from build123d import *

# Parameters (mm, degrees)
BOSS_EXTRUDE3_DEPTH      = 3.249999
BOSS_EXTRUDE3_DEPTH_BACK = 16.581442
SKETCH1_W                = 34.3
SKETCH1_H                = 66.5
CUT_EXTRUDE1_DEPTH       = 5
CUT_EXTRUDE2_DEPTH       = 5
FILLET1_R                = 2
SKETCH5_W                = 51.30778099
SKETCH5_H                = 76.39990746
CUT_EXTRUDE3_DEPTH       = 14
SKETCH6_W                = 31.3
SKETCH6_H                = 63.5
CUT_EXTRUDE4_DEPTH       = 4.831437303
SKETCH7_W                = 26.3
SKETCH7_H                = 4
SKETCH7_W_2              = 25.3
BOSS_EXTRUDE4_DEPTH      = 9.5
SKETCH8_W                = 20.3
SKETCH8_H                = 55.5
BOSS_EXTRUDE5_DEPTH      = 2
CUT_EXTRUDE5_DEPTH       = 1.5


with BuildPart() as part:
    # Sketch1 → Boss-Extrude3 (new, two sides: drawn at the far end of the back side and taken through both)
    with BuildSketch(Plane.XY.offset(-BOSS_EXTRUDE3_DEPTH_BACK)):
        with Locations((-15.15, 31.25)):
            Rectangle(SKETCH1_W, SKETCH1_H)
    extrude(amount=BOSS_EXTRUDE3_DEPTH + BOSS_EXTRUDE3_DEPTH_BACK)

    # Sketch3 → Cut-Extrude1 (cut)
    with BuildSketch(Plane.ZY.offset(32.3)):
        with BuildLine():
            Line((-13.946442816, 47.860002379), (-13.946442816, 14.260002379))
            add(Edge.make_bspline(
                [(-13.946442816, 14.260002379), (-13.946442816, 14.019317473), (-13.90167089, 13.549905983), (-13.594210712, 12.544215416), (-12.741245974, 11.38215204), (-11.448721179, 10.74393594), (-10.404919412, 10.615783107), (-9.934864774, 10.653203818), (-9.697836412, 10.694998313)],
                knots=[0, 0, 0, 0, 0.125, 0.25, 0.5, 0.75, 0.875, 1, 1, 1, 1], degree=3))
            Line((-9.697836412, 10.694998313), (-6.707836413, 11.222215985))
            add(Edge.make_bspline(
                [(-6.707836413, 11.222215985), (-6.30796959, 11.292723295), (-5.54451734, 11.557407058), (-4.497780226, 12.405299319), (-3.844533346, 13.58336909), (-3.716442816, 14.381184638), (-3.716442816, 14.787220052)],
                knots=[0, 0, 0, 0, 0.25, 0.5, 0.75, 1, 1, 1, 1], degree=3))
            Line((-3.716442816, 14.787220052), (-3.716442816, 47.332784706))
            add(Edge.make_bspline(
                [(-3.716442816, 47.332784706), (-3.716442815, 47.73882012), (-3.844533346, 48.536635667), (-4.497780225, 49.714705439), (-5.544517339, 50.5625977), (-6.307969589, 50.827281463), (-6.707836412, 50.897788773)],
                knots=[0, 0, 0, 0, 0.25, 0.5, 0.75, 1, 1, 1, 1], degree=3))
            Line((-6.707836412, 50.897788773), (-9.697836412, 51.425006445))
            add(Edge.make_bspline(
                [(-9.697836412, 51.425006445), (-9.934864773, 51.46680094), (-10.404919411, 51.504221651), (-11.448721179, 51.376068818), (-12.741245974, 50.737852719), (-13.594210712, 49.575789343), (-13.90167089, 48.570098776), (-13.946442816, 48.100687285), (-13.946442816, 47.860002379)],
                knots=[0, 0, 0, 0, 0.125, 0.25, 0.5, 0.75, 0.875, 1, 1, 1, 1], degree=3))
        make_face()
    extrude(amount=-CUT_EXTRUDE1_DEPTH, mode=Mode.SUBTRACT)

    # Sketch4 → Cut-Extrude2 (cut)
    with BuildSketch(Plane(origin=(2, 0, 0), x_dir=(0, 0, -1), z_dir=(1, 0, 0))):
        with BuildLine():
            Line((6.817836087, 38.212213104), (9.807836086, 37.684995431))
            add(Edge.make_bspline(
                [(9.807836086, 37.684995431), (10.044864448, 37.643200936), (10.514919086, 37.605780225), (11.558720853, 37.733933058), (12.851245648, 38.372149158), (13.704210386, 39.534212534), (14.011670565, 40.539903101), (14.05644249, 41.009314591), (14.05644249, 41.249999497)],
                knots=[0, 0, 0, 0, 0.125, 0.25, 0.5, 0.75, 0.875, 1, 1, 1, 1], degree=3))
            Line((14.05644249, 41.249999497), (14.05644249, 52.799999497))
            add(Edge.make_bspline(
                [(14.05644249, 52.799999497), (14.05644249, 53.040684403), (14.011670565, 53.510095894), (13.704210386, 54.51578646), (12.851245648, 55.677849837), (11.558720853, 56.316065936), (10.514919086, 56.444218769), (10.044864448, 56.406798058), (9.807836087, 56.365003563)],
                knots=[0, 0, 0, 0, 0.125, 0.25, 0.5, 0.75, 0.875, 1, 1, 1, 1], degree=3))
            Line((9.807836087, 56.365003563), (6.817836087, 55.837785891))
            add(Edge.make_bspline(
                [(6.817836087, 55.837785891), (6.417969263, 55.767278581), (5.654517014, 55.502594818), (4.6077799, 54.654702557), (3.95453302, 53.476632786), (3.82644249, 52.678817239), (3.82644249, 52.272781825)],
                knots=[0, 0, 0, 0, 0.25, 0.5, 0.75, 1, 1, 1, 1], degree=3))
            Line((3.82644249, 52.272781825), (3.82644249, 41.77721717))
            add(Edge.make_bspline(
                [(3.82644249, 41.77721717), (3.82644249, 41.371181756), (3.95453302, 40.573366208), (4.6077799, 39.395296437), (5.654517014, 38.547404177), (6.417969263, 38.282720413), (6.817836087, 38.212213104)],
                knots=[0, 0, 0, 0, 0.25, 0.5, 0.75, 1, 1, 1, 1], degree=3))
        make_face()
        with BuildLine():
            Line((3.82644249, 20.772783732), (3.82644249, 10.277219077))
            add(Edge.make_bspline(
                [(3.82644249, 10.277219077), (3.82644249, 9.871183663), (3.95453302, 9.073368116), (4.6077799, 7.895298345), (5.654517014, 7.047406084), (6.417969263, 6.782722321), (6.817836087, 6.712215011)],
                knots=[0, 0, 0, 0, 0.25, 0.5, 0.75, 1, 1, 1, 1], degree=3))
            Line((6.817836087, 6.712215011), (9.807836086, 6.184997339))
            add(Edge.make_bspline(
                [(9.807836086, 6.184997339), (10.044864448, 6.143202843), (10.514919086, 6.105782132), (11.558720853, 6.233934965), (12.851245648, 6.872151065), (13.704210386, 8.034214441), (14.011670565, 9.039905008), (14.05644249, 9.509316499), (14.05644249, 9.750001404)],
                knots=[0, 0, 0, 0, 0.125, 0.25, 0.5, 0.75, 0.875, 1, 1, 1, 1], degree=3))
            Line((14.05644249, 9.750001404), (14.05644249, 21.300001404))
            add(Edge.make_bspline(
                [(14.05644249, 21.300001404), (14.05644249, 21.54068631), (14.011670565, 22.010097801), (13.704210386, 23.015788368), (12.851245648, 24.177851744), (11.558720853, 24.816067843), (10.514919086, 24.944220677), (10.044864448, 24.906799966), (9.807836087, 24.86500547)],
                knots=[0, 0, 0, 0, 0.125, 0.25, 0.5, 0.75, 0.875, 1, 1, 1, 1], degree=3))
            Line((9.807836087, 24.86500547), (6.817836087, 24.337787798))
            add(Edge.make_bspline(
                [(6.817836087, 24.337787798), (6.417969263, 24.267280488), (5.654517014, 24.002596725), (4.6077799, 23.154704464), (3.95453302, 21.976634693), (3.82644249, 21.178819146), (3.82644249, 20.772783732)],
                knots=[0, 0, 0, 0, 0.25, 0.5, 0.75, 1, 1, 1, 1], degree=3))
        make_face()
    extrude(amount=-CUT_EXTRUDE2_DEPTH, mode=Mode.SUBTRACT)

    # Fillet1
    fillet1_edges = [part.edges().sort_by_distance(p)[0] for p in [
        (-32.3, -2, -6.6657215),
        (2, -2, -6.6657215),
        (2, 64.5, -6.6657215),
        (-32.3, 64.5, -6.6657215),
    ]]
    fillet(fillet1_edges, radius=FILLET1_R)

    # Sketch5 → Cut-Extrude3 (cut)
    with BuildSketch(Plane(origin=(0, 2.84e-07, 3.250003097), x_dir=(1, 0, 0), z_dir=(0, 8.742273400000003e-08, 0.9999999999999963))):
        with Locations((-12.815688561, 29.564706803)):
            Rectangle(SKETCH5_W, SKETCH5_H)
    extrude(amount=-CUT_EXTRUDE3_DEPTH, mode=Mode.SUBTRACT)


with BuildPart() as cut_extrude3_kept_piece:
    # of the separate pieces the step leaves, the one the design keeps (cut_extrude3_pieces_kept)
    add(part.part.solids().sort_by_distance((-30.3, 64.5, -16.581442))[0])

    # Sketch6 → Cut-Extrude4 (cut)
    with BuildSketch(Plane(origin=(0, -9.4e-07, -10.749996903), x_dir=(1, 0, 0), z_dir=(0, 8.742273399652584e-08, 0.9999999999999963))):
        with Locations((-15.15, 31.25000094)):
            Rectangle(SKETCH6_W, SKETCH6_H)
    extrude(amount=-CUT_EXTRUDE4_DEPTH, mode=Mode.SUBTRACT)


with BuildPart() as boss_extrude4_tool:
    # Sketch7 → Boss-Extrude4 (new body)
    with BuildSketch(Plane(origin=(1.362e-06, 0, -15.581439757), x_dir=(0.9999999999999963, 0, 8.742273400000003e-08), z_dir=(-8.742273400000003e-08, 1.0000000000000005e-15, 0.9999999999999963))):
        with Locations((-17.650001362, 60.999999578)):
            Rectangle(SKETCH7_W, SKETCH7_H)
        with Locations((-18.150001362, 1.499999578)):
            Rectangle(SKETCH7_W_2, SKETCH7_H)
    extrude(amount=BOSS_EXTRUDE4_DEPTH)


with BuildPart() as cut_extrude3_kept_piece_1:
    add(cut_extrude3_kept_piece.part)


with BuildPart() as cut_extrude3_kept_piece_2:
    # Boss-Extrude4: joined with boss_extrude4_tool
    add(cut_extrude3_kept_piece_1.part.fuse(boss_extrude4_tool.part, tol=0.00001))

    # Sketch8 → Boss-Extrude5 (add)
    with BuildSketch(Plane(origin=(1.362e-06, 0, -15.581439757), x_dir=(0.9999999999999963, 0, 8.742273400000003e-08), z_dir=(-8.742273400000003e-08, 1.0000000000000005e-15, 0.9999999999999963))):
        with Locations((-14.650001362, 31.249999578)):
            Rectangle(SKETCH8_W, SKETCH8_H)
    extrude(amount=BOSS_EXTRUDE5_DEPTH)

    # Sketch9 → Cut-Extrude5 (cut)
    with BuildSketch(Plane.ZY.offset(32.3)):
        with BuildLine():
            Line((-11.974063023, 54.635108256), (-11.974063023, 7.533043045))
            ThreePointArc((-11.974063023, 7.533043045), (-8.974063023, 4.533043045), (-5.974063023, 7.533043045))
            Line((-5.974063023, 7.533043045), (-5.974063023, 54.635108256))
            ThreePointArc((-5.974063023, 54.635108256), (-8.974063023, 57.635108256), (-11.974063023, 54.635108256))
        make_face()
    extrude(amount=-CUT_EXTRUDE5_DEPTH, mode=Mode.SUBTRACT)


solid = cut_extrude3_kept_piece_2.part
Check sheet for the modelled part. Datum: model origin and axes. Units: mm. A direction names the side the tool comes from. Round coordinates to 2 decimals unless told otherwise and drop trailing zeros. Order: outer loops, then holes, each group sorted by start corner. A loop starts at its lowest first (then second) coordinate and runs counter-clockwise, first axis right, second up. Notation, with made-up numbers: M 35,31.5 L 50,31.5 A33 cw 50,69.5 Z; hole C 3.25,45.25 d3. An arc over 180 degrees is marked long. One line per item, written item: value. Start each with the question number.
1. Access from +Z, -Z, +X, -X, +Y, -Y to the whole of each face (thin tool, end or side, straight path). Record for faces 4 (the flat face through (-15, 32, -13.581)), 5 (the flat face through (-18, -0.5, -8)), 6 (the cylindrical face through (-31.56, 6.2, -11.66)), 7 (the flat face through (1, 47, -14.056)), 8 (the flat face through (-32, 53, -11.974)).
2. Section check C-C on x = -2.5. Enter the section's corners in (y, z).
3. Release check for a two-part mould opening along Y. For faces 1 (the flat face through (-18, 2, -6.081)), 2 (the flat face through (-32, 9, -11.974)), 3 (the flat face through (-15, 64.5, -14)) record: released by +Y, released by -Y, zero draft, split by the parting line, or undercut.
4. Section check A-A on z = -7.5. Enter the section's corners in (x, y), and give its area (3 significant figures).
5. Section check B-B on y = 60.5. Enter the section's corners in (x, z), and give its area (3 significant figures).
6. Scan lines: line 1 along X through (y, z) = (53.5, -15); line 2 along Y through (x, z) = (-17, -8); line 3 along Y through (x, z) = (-4, -14). Record each from-to range of solid material in increasing order.
7. Section check D-D on z = -12.75. Give the number of separate pieces and of enclosed holes in the cut face, and give its area (3 significant figures).
8. Gauge pin test, flat ends, axial feed: P1, Ø10, axis at x = -26, y = 29, coming from the +Z side; P2, Ø12, axis at x = -4.5, y = 29.5, coming from the +Z side; P3, Ø2.5, axis at x = -16, z = -9, coming from the +Y side. Record the tip position at first contact, or that the pin passes through.
Results found:
1. face 4: +Z
1. face 5: +Z, +X, -X, -Y
1. face 6: +Z, -X
1. face 7: +Z, +X
1. face 8: +Z, +X, -X
2. outline: M -2,-16.58 L 64.5,-16.58 L 64.5,-10.75 L 63,-10.75 L 63,-15.58 L -0.5,-15.58 L -0.5,-10.75 L -2,-10.75 Z
3. face 1: zero draft
3. face 2: undercut
3. face 3: released by +Y
4. outline: M -30.8,-0.5 L -5.5,-0.5 L -5.5,3.5 L -30.8,3.5 Z; M -30.8,59 L -4.5,59 L -4.5,63 L -30.8,63 Z
4. area: 206 mm^2
5. outline: M -32.3,-16.58 L 2,-16.58 L 2,-10.75 L 0.5,-10.75 L 0.5,-15.58 L -4.5,-15.58 L -4.5,-6.08 L -30.8,-6.08 L -30.8,-10.75 L -32.3,-10.75 Z
5. area: 299 mm^2
6. line 1: -32.3 to -30.8, -24.8 to -4.5, 0.5 to 2
6. line 2: -0.5 to 3.5, 59 to 63
6. line 3: -2 to -0.5, 63 to 64.5
7. separate pieces: 3
7. enclosed holes: 0
7. area: 387 mm^2
8. P1: z = -13.58
8. P2: z = -10.75
8. P3: y = 63
